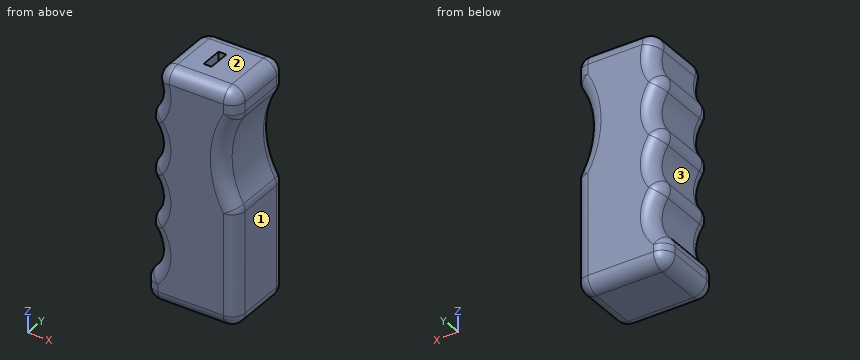
from build123d import *

# Parameters (mm, degrees)
F0_W     = 35
F0_H     = 90
F1_DEPTH = 27.94
F3_DEPTH = 27.941
F4_W     = 3
F4_H     = 8.5
F5_DEPTH = 30
F6_R     = 5


with BuildPart() as f1:
    # F0 (on Front) → F1 (new body)
    with BuildSketch(Plane.XZ):
        with Locations((17.5, 45)):
            Rectangle(F0_W, F0_H)
    extrude(amount=F1_DEPTH)

    # F2 (on face) → F3 (cut, through all)
    with BuildSketch(Plane.XZ.offset(27.94)):
        with BuildLine():
            Line((35, 45), (35, 80))
            ThreePointArc((35, 80), (30, 62.5), (35, 45))
        make_face()
        with BuildLine():
            ThreePointArc((0, 70), (5, 80), (0, 90))
            Line((0, 90), (0, 70))
        make_face()
        with BuildLine():
            ThreePointArc((0, 50), (5, 60), (0, 70))
            Line((0, 70), (0, 50))
        make_face()
        with BuildLine():
            ThreePointArc((0, 30), (5, 40), (0, 50))
            Line((0, 50), (0, 30))
        make_face()
        with BuildLine():
            Line((0, 30), (0, 10))
            ThreePointArc((0, 10), (5, 20), (0, 30))
        make_face()
    extrude(amount=-F3_DEPTH, mode=Mode.SUBTRACT)

    # F4 (on face) → F5 (cut)
    with BuildSketch(Plane.XY.offset(90)):
        with Locations((17.5, -13.97)):
            Rectangle(F4_W, F4_H)
    extrude(amount=-F5_DEPTH, mode=Mode.SUBTRACT)

    # F6
    f6_edges = [f1.edges().sort_by_distance(p)[0] for p in [
        (5, -27.94, 60),
        (0, -13.97, 70),
        (5, 0, 60),
        (0, -13.97, 50),
        (5, -27.94, 80),
        (0, -13.97, 90),
        (5, 0, 80),
        (5, 0, 40),
        (5, -27.94, 40),
        (0, 0, 5),
        (0, -13.97, 0),
        (0, -27.94, 5),
        (0, -13.97, 10),
        (35, -13.97, 0),
        (17.5, 0, 0),
        (17.5, -27.94, 0),
        (35, 0, 22.5),
        (35, -13.97, 45),
        (35, -27.94, 22.5),
        (30, -27.94, 62.5),
        (30, 0, 62.5),
        (35, -13.97, 80),
        (35, 0, 85),
        (35, -13.97, 90),
        (35, -27.94, 85),
        (17.5, 0, 90),
        (17.5, -27.94, 90),
        (5, -27.94, 20),
        (5, 0, 20),
        (0, -13.97, 30),
    ]]
    fillet(f6_edges, radius=F6_R)


solid = f1.part
Could you check a few things on this model? Use its own coordinates, in mm. Face numbers are marked on the shaded views. Give positions to 0.01 mm unless a question says otherwise; leave off trailing zeros. Order: outer loops, then holes, each group sorted by start corner. A loop starts at its lowest first (then second) coordinate and runs counter-clockwise, first axis right, second up. Notation, with made-up numbers: (68, 63.25) - (72, 63.25) arc R13 ccw to (72, 88.25) - close; hole circle Ø9 at (74, 42). An arc over 180 degrees is marked (long way). One line per question, with ' | ' between items. Start each with the question number.
Item 1: I'm going to push flat-ended pins straight in: pin 1 Ø1 at (y, z) = (-24, 10.5) entering from +X; pin 2 Ø6 at (y, z) = (-15, 69) entering from +X; pin 3 Ø2.5 at (y, z) = (-12.5, 71) entering from -X. Where does each tip first touch, or does it pass through?
Item 2: I want a section at C-C on y = -3. Write out the boundary of the cut face in (x, z) (1 decimal).
Item 3: I need wall thicknesses on probe 1 along X at (y, z) = (-13, 30); probe 2 along Y at (x, z) = (8.5, 13.5); probe 3 along Z at (x, y) = (17.5, -15.25). Which ranges of each line are inside material? Lowest first, please. Write a range as [from, to].
Item 4: I want a section at A-A on x = 18. Write out the boundary of the cut face in (y, z).
Item 5: I want a section at B-B on y = -25.5. Write out the boundary of the cut face in (x, z) (1 decimal).
Item 6: Thinking about a two-plate mould opening in Z: for the marked faces 1, 2 and 3, which applies, pulls with the +Z half, pulls with the -Z half, needs draft (parallel to the pull), parting line crosses it, or undercut?
Verdict:
1) pin 1: x = 34.97 | pin 2: x = 31.39 | pin 3: x = 1.86
2) outline: (0.4, 5) arc R4.6 ccw to (5, 0.4) - (30, 0.4) arc R4.6 ccw to (34.6, 5) - (34.6, 43.6) arc R4.6 ccw to (34, 45.9) arc R33.5 cw to (34, 79.1) arc R4.6 ccw to (34.6, 81.4) - (34.6, 85) arc R4.6 ccw to (30, 89.6) - (9.3, 89.6) arc R4.6 ccw to (4.9, 83.7) arc R12.9 cw to (3.1, 72.6) arc R4.6 ccw to (3.1, 67.4) arc R12.9 cw to (3.1, 52.6) arc R4.6 ccw to (3.1, 47.4) arc R12.9 cw to (3.1, 32.6) arc R4.6 ccw to (3.1, 27.4) arc R12.9 cw to (1.7, 11) arc R4.6 ccw to (0.4, 7.8) - close
3) probe 1: [1.86, 35] | probe 2: [-27.93, -0.01] | probe 3: [0, 60]
4) outline: (-27.94, 5) arc R5 ccw to (-22.94, 0) - (-5, 0) arc R5 ccw to (0, 5) - (0, 85) arc R5 ccw to (-5, 90) - (-9.72, 90) - (-9.72, 60) - (-18.22, 60) - (-18.22, 90) - (-22.94, 90) arc R5 ccw to (-27.94, 85) - close
5) outline: (0.7, 5) arc R4.3 ccw to (5, 0.7) - (30, 0.7) arc R4.3 ccw to (34.3, 5) - (34.3, 43.6) arc R4.3 ccw to (33.7, 45.8) arc R33.8 cw to (33.7, 79.2) arc R4.3 ccw to (34.3, 81.4) - (34.3, 85) arc R4.3 ccw to (30, 89.3) - (9.3, 89.3) arc R4.3 ccw to (5.2, 83.8) arc R13.2 cw to (3.3, 72.5) arc R4.3 ccw to (3.3, 67.5) arc R13.2 cw to (3.3, 52.5) arc R4.3 ccw to (3.3, 47.5) arc R13.2 cw to (3.3, 32.5) arc R4.3 ccw to (3.3, 27.5) arc R13.2 cw to (1.9, 10.8) arc R4.3 ccw to (0.7, 7.8) - close
6) face 1: needs draft | face 2: pulls with the +Z half | face 3: undercut
